The figure shows three views and two pictorial views of one solid part (mm, origin at its lowest corner). Answer the questions. Round coordinates to 2 decimals unless told otherwise and drop trailing zeros. Write each loop counter-clockwise with the first axis right and the second up, starting at its lowest first coordinate (ties: lowest second). Pieces come first, ordered by that corner, then holes. Notation, with made-up numbers: M -5,-0.75 L 6,-0.75 A25 ccw 6,34.25 Z; hole C 81,26 d2. An arc over 180 degrees is marked long. Answer in a Markdown table with one row per item.
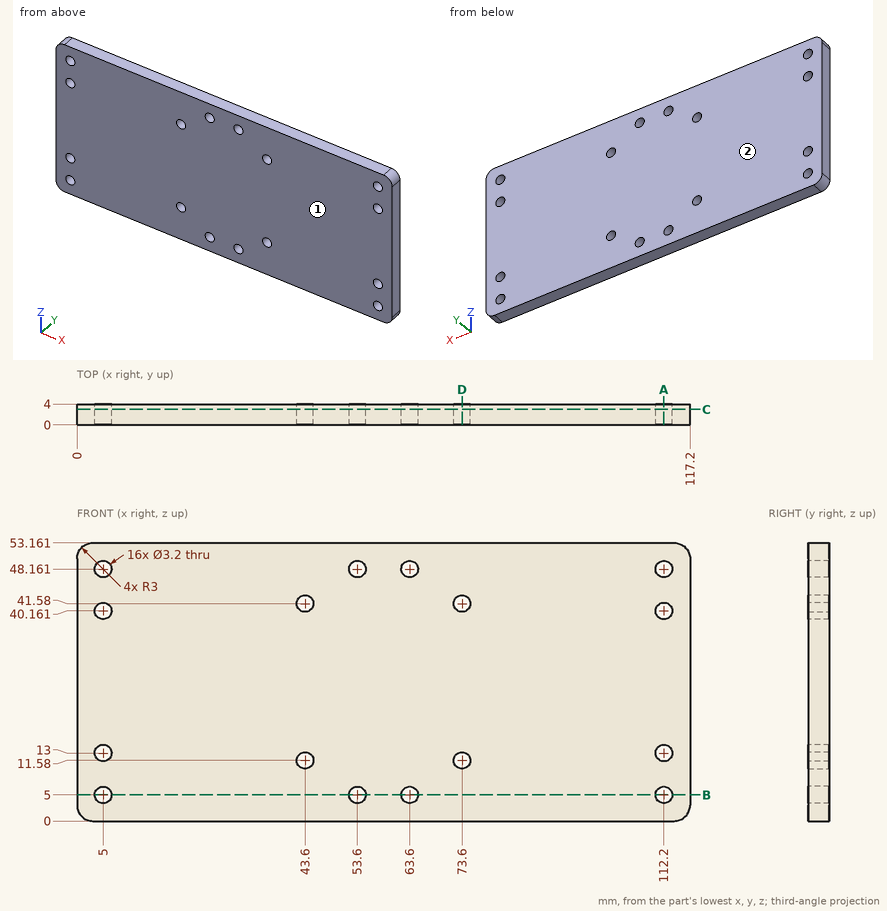
1. Consider line 1 along Z through (x, y) = (63.5, 1.4); line 2 along X through (y, z) = (2.4, 12.5); line 3 along X through (y, z) = (2.9, 13) (1 decimal). Determine where each line is inside the solid, lowest interval first. Write a range as from..to.
Calculated:
| item | result |
|---|---|
| line 1 | z = 0..3.4, 6.6..46.56, 49.76..53.16 |
| line 2 | x = 0..3.48, 6.52..42.29, 44.91..72.29, 74.91..110.68, 113.72..117.2 |
| line 3 | x = 0..3.4, 6.6..42.9, 44.3..72.9, 74.3..110.6, 113.8..117.2 |
2. Determine the mould class of the marked faces 1 and 2 for opening direction Y: released by +Y, released by -Y, zero draft, split by the parting line, or undercut.
Calculated:
| item | result |
|---|---|
| face 1 | released by -Y |
| face 2 | released by +Y |
3. The part is cut by section C-C (y = 2.95). Count the separate pieces of the cut face and the enclosed holes in it, plus the area to 3 significant figures.
Calculated:
| item | result |
|---|---|
| separate pieces | 1 |
| enclosed holes | 16 |
| area | 6,090 mm² |
4. The part is cut by section A-A (x = 112.2). Determine the outline of the cut face in (y, z).
Calculated:
| item | result |
|---|---|
| outline | M 0,0 L 4,0 L 4,3.4 L 0,3.4 Z; M 0,6.6 L 4,6.6 L 4,11.4 L 0,11.4 Z; M 0,14.6 L 4,14.6 L 4,38.56 L 0,38.56 Z; M 0,41.76 L 4,41.76 L 4,46.56 L 0,46.56 Z; M 0,49.76 L 4,49.76 L 4,53.16 L 0,53.16 Z |
5. The part is cut by section D-D (x = 73.6). Determine the outline of the cut face in (y, z).
Calculated:
| item | result |
|---|---|
| outline | M 0,0 L 4,0 L 4,9.98 L 0,9.98 Z; M 0,13.18 L 4,13.18 L 4,39.98 L 0,39.98 Z; M 0,43.18 L 4,43.18 L 4,53.16 L 0,53.16 Z |
6. The part is cut by section B-B (z = 5). Determine the outline of the cut face in (x, y).
Calculated:
| item | result |
|---|---|
| outline | M 0,0 L 3.4,0 L 3.4,4 L 0,4 Z; M 6.6,0 L 52,0 L 52,4 L 6.6,4 Z; M 55.2,0 L 62,0 L 62,4 L 55.2,4 Z; M 65.2,0 L 110.6,0 L 110.6,4 L 65.2,4 Z; M 113.8,0 L 117.2,0 L 117.2,4 L 113.8,4 Z |
